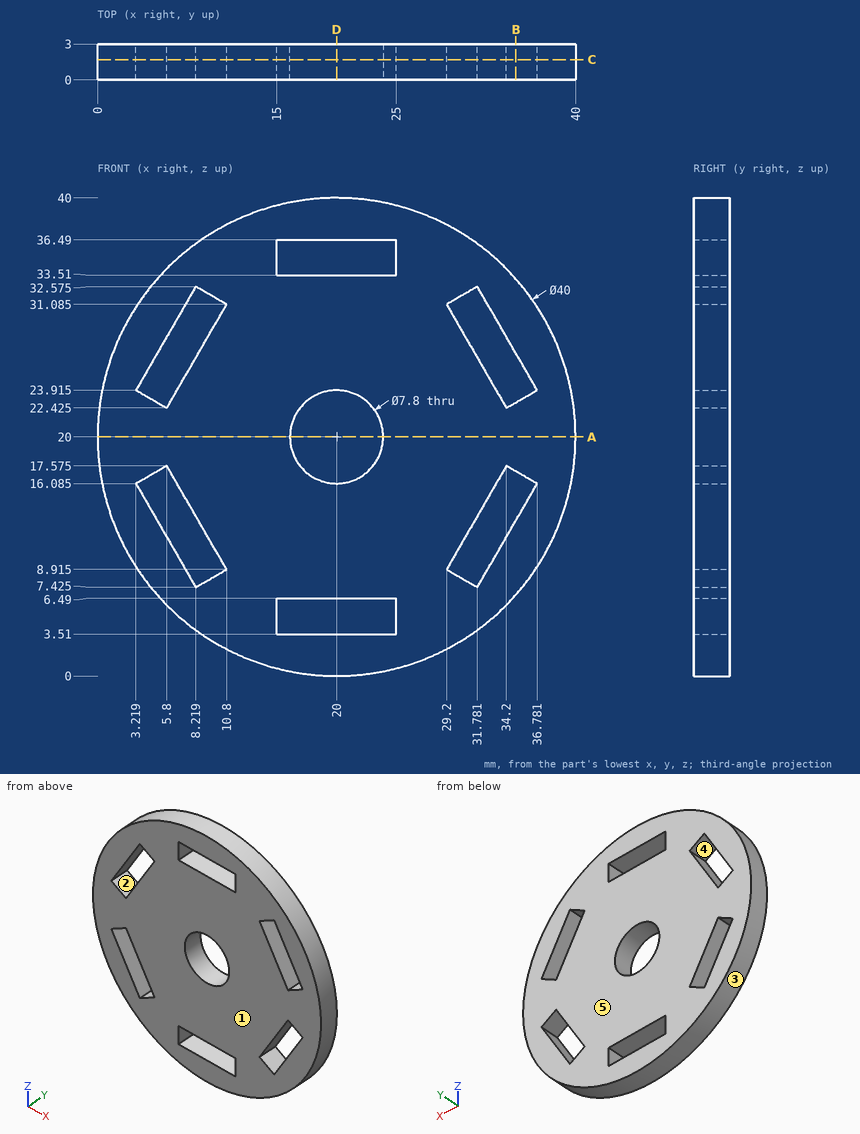
Geometry check sheet. Reference: drawing and pictorial views, mm from the part's lowest x, y, z. A direction names the side the tool comes from. Round coordinates to 2 decimals unless told otherwise and drop trailing zeros. Order: outer loops, then holes, each group sorted by start corner. A loop starts at its lowest first (then second) coordinate and runs counter-clockwise, first axis right, second up. Notation, with made-up numbers: (21, 29.25) - (71, 29.25) arc R27 cw to (71, 57.25) - close; hole circle Ø2 at (32.5, -26). An arc over 180 degrees is marked (long way). Use a Markdown table: item, result. Add a question column.
1) Mould release check, pull along Z, two halves, no side actions. Record for the marked faces 1, 2 and 3: released by +Z, released by -Z, zero draft, split by the parting line, or undercut.
2) Section check D-D (x = 20). Record the cut outline in (y, z).
3) Set-up check for the marked faces 4 and 5: record each of +Z, -Z, +X, -X, +Y, -Y from which the full face is reachable in a straight line by a thin tool's end or side.
4) Section check C-C (y = 1.7). Record the cut outline in (x, z) (1 decimal).
5) Thickness scan on line 1 along Z through (x, y) = (20, 1.4); line 2 along X through (y, z) = (1.35, 31.5) (1 decimal); line 3 along X through (y, z) = (0.1, 31). Record the ranges inside material, lowest first.
6) Gauge pin test, flat ends, axial feed: P1, Ø1.5, axis at y = 0.5, z = 8.5, coming from the -X side (1 decimal); P2, Ø0.9, axis at x = 19, y = 1, coming from the -Z side; P3, Ø1.5, axis at y = 1.5, z = 35.5, coming from the +X side. Record the tip position at first contact, or that the pin passes through.
7) Section check B-B (x = 35). Record the cut outline in (y, z).
8) Section check A-A (z = 20). Record the cut outline in (x, y).
Established:
| question | item | result |
|---|---|---|
| 1 | face 1 | zero draft |
| 1 | face 2 | undercut |
| 1 | face 3 | split by the parting line |
| 2 | outline | (0, 0) - (3, 0) - (3, 3.51) - (0, 3.51) - close; (0, 6.49) - (3, 6.49) - (3, 16.1) - (0, 16.1) - close; (0, 23.9) - (3, 23.9) - (3, 33.51) - (0, 33.51) - close; (0, 36.49) - (3, 36.49) - (3, 40) - (0, 40) - close |
| 3 | face 4 | +Y, -Y |
| 3 | face 5 | +Z, -Z, +X, -X, +Y |
| 4 | outline | circle Ø40 at (20, 20); hole (3.2, 16.1) - (8.2, 7.4) - (10.8, 8.9) - (5.8, 17.6) - close; hole (3.2, 23.9) - (5.8, 22.4) - (10.8, 31.1) - (8.2, 32.6) - close; hole (15, 3.5) - (25, 3.5) - (25, 6.5) - (15, 6.5) - close; hole (15, 33.5) - (25, 33.5) - (25, 36.5) - (15, 36.5) - close; hole circle Ø7.8 at (20, 20); hole (29.2, 8.9) - (31.8, 7.4) - (36.8, 16.1) - (34.2, 17.6) - close; hole (29.2, 31.1) - (34.2, 22.4) - (36.8, 23.9) - (31.8, 32.6) - close |
| 5 | line 1 | 0 to 3.51, 6.49 to 16.1, 23.9 to 33.51, 36.49 to 40 |
| 5 | line 2 | 3.6 to 7.6, 10.1 to 29.9, 32.4 to 36.4 |
| 5 | line 3 | 3.3 to 7.31, 10.75 to 29.25, 32.69 to 36.7 |
| 6 | P1 | x = 3.1 |
| 6 | P2 | z = 0.01 |
| 6 | P3 | x = 33.51 |
| 7 | outline | (0, 6.77) - (3, 6.77) - (3, 13) - (0, 13) - close; (0, 17.11) - (3, 17.11) - (3, 22.89) - (0, 22.89) - close; (0, 27) - (3, 27) - (3, 33.23) - (0, 33.23) - close |
| 8 | outline | (0, 0) - (16.1, 0) - (16.1, 3) - (0, 3) - close; (23.9, 0) - (40, 0) - (40, 3) - (23.9, 3) - close |
